Work out the finished part from the listing and answer in its coordinate system (mm). Face numbers are marked on the shaded views. A direction names the side the tool comes from. Coordinates: 2 decimals unless noted, no trailing zeros. Loops run counter-clockwise (first coordinate to the right, second up) from the corner with the lowest first, then second, coordinate; pieces in that order, holes last. Notation, with made-up numbers: (0, 61) - (31, 61) arc R7 cw to (31, 72) - close; hole circle Ø2 at (15.25, 89). An arc over 180 degrees is marked (long way). Write each question's results on one line, items separated by ' | '. Start each with the question number.
Item 1: A tool of negligible diameter and unlimited length cuts with its end or side. For the marked faces 5, 6, 7, 8 and 9, from which of +Z, -Z, +X, -X, +Y, -Y can it reach the whole face along a straight path? Write none if from no direction.
Item 2: Each of these flat-tipped pins is pushed along its axis until it touches: pin 1 Ø2 at (x, y) = (-15.5, 32.5) entering from -Z; pin 2 Ø5.5 at (x, z) = (6.5, -2) entering from +Y; pin 3 Ø2 at (x, y) = (-17, 32) entering from +Z. Where does it stop, or does it pass through?
Item 3: Section A-A, the plane y = 9 is taken. Write down the section's boundary in (x, z), plus the area to 3 significant figures.
Item 4: Consider probe 1 along X at (y, z) = (35, -1.5); probe 2 along X at (y, z) = (-2, 2); probe 3 along Z at (x, y) = (-4.5, -16). Determine where each line is inside the solid, lowest interval first. Write a range as [from, to].
Item 5: For a pull along Y with two mould halves and no side action, classify the marked faces 1, 2, 3 and 4 as +Y half, -Y half, draft (parallel to the pull), parting line (faces both ways), or undercut.
from build123d import *

# Parameters (mm, degrees)
SKETCH2_R           = 3.96875
BOSS_EXTRUDE1_DEPTH = 34.925
CHAMFER2_SIZE       = 1.058333333
SKETCH7_R           = 3.96875
SKETCH9_R           = 3.96875
BOSS_EXTRUDE2_DEPTH = 3.3734375
SKETCH10_OUTSIDE_W  = 257.161
SKETCH10_OUTSIDE_H  = 225.222
SKETCH10_OUTSIDE_R  = 6.35
CUT_EXTRUDE1_DEPTH  = 56.231770933
CUT_EXTRUDE1_TAPER  = 60
SKETCH11_OUTSIDE_W  = 117.847
SKETCH11_OUTSIDE_H  = 85.908
SKETCH11_OUTSIDE_R  = 6.35
CUT_EXTRUDE2_DEPTH  = 16.015104167
CUT_EXTRUDE2_TAPER  = 60
SKETCH12_W          = 52.3875
SKETCH12_H          = 19.05
BOSS_EXTRUDE3_DEPTH = 2.38125


with BuildPart() as part:
    # Sketch2 → Boss-Extrude1 (new body)
    with BuildSketch(Plane(origin=(0, 42.8625, 0), x_dir=(-1, 0, 0), z_dir=(0, 1, 0))):
        with Locations((16.66875, 0)):
            Circle(SKETCH2_R)
    extrude(amount=-BOSS_EXTRUDE1_DEPTH)

    # Chamfer2
    chamfer2_edges = [part.edges().sort_by_distance(p)[0] for p in [
        (-12.7, 42.8625, 0),
    ]]
    chamfer(chamfer2_edges, length=CHAMFER2_SIZE)


with BuildPart() as body_2:
    # Sweep1: sweep along a path in Sketch8
    with BuildLine(Plane.XY) as sweep1_path:
        Line((-16.66875, 7.9375), (-16.66875, 0))
        ThreePointArc((-16.66875, 0), (0, -16.66875), (16.66875, 0))
        Line((16.66875, 0), (16.66875, 7.9375))
    # Sketch7 → Sweep1 (sweep)
    with BuildSketch(Plane(origin=(0, 7.9375, 0), x_dir=(-1, 0, 0), z_dir=(0, 1, 0))):
        with Locations((16.66875, 0)):
            Circle(SKETCH7_R)
    sweep(path=sweep1_path.line)


with BuildPart() as body_3:
    # Body-Move/Copy1: copy of part
    add(part.part.moved(Location((33.3375, 0, 0))))


with BuildPart() as part_1:
    add(part.part)

    # Combine1: union body 2, body 3
    add(body_2.part)
    add(body_3.part)



with BuildPart() as body_2_2:
    # Sketch9 → Boss-Extrude2 (new body, symmetric)
    with BuildSketch(Plane(origin=(0, 31.220833333, 0), x_dir=(-1, 0, 0), z_dir=(0, 1, 0))):
        Polygon((-20.334924209, 6.35), (-24.001098419, 0), (-20.334924209, -6.35), (-13.002575791, -6.35), (-9.336401581, 0), (-13.002575791, 6.35), align=None)
        with Locations((-16.66875, 0)):
            Circle(SKETCH9_R, mode=Mode.SUBTRACT)
    extrude(amount=BOSS_EXTRUDE2_DEPTH, both=True)

    # Sketch10 outside → Cut-Extrude1 (cut, through all)
    with BuildSketch(Plane(origin=(0, 34.594270833, 0), x_dir=(1, 0, 0), z_dir=(0, 1, 0))):
        with Locations((1.6815, 0)):
            Rectangle(SKETCH10_OUTSIDE_W, SKETCH10_OUTSIDE_H)
        with Locations((16.66875, 0)):
            Circle(SKETCH10_OUTSIDE_R, mode=Mode.SUBTRACT)
    extrude(amount=-CUT_EXTRUDE1_DEPTH, taper=CUT_EXTRUDE1_TAPER, mode=Mode.SUBTRACT)

    # Sketch11 outside → Cut-Extrude2 (cut, through all)
    with BuildSketch(Plane.XZ.offset(-27.847395833)):
        with Locations((1.6815, 0)):
            Rectangle(SKETCH11_OUTSIDE_W, SKETCH11_OUTSIDE_H)
        with Locations((16.66875, 0)):
            Circle(SKETCH11_OUTSIDE_R, mode=Mode.SUBTRACT)
    extrude(amount=-CUT_EXTRUDE2_DEPTH, taper=CUT_EXTRUDE2_TAPER, mode=Mode.SUBTRACT)


with BuildPart() as body_3_2:
    # Body-Move/Copy2: copy of body 2 2
    add(body_2_2.part.moved(Location((-33.3375, 0, 0))))


with BuildPart() as part_2:
    add(part_1.part)

    add(body_2_2.part)  # Boss-Extrude3 merges body 2 2

    add(body_3_2.part)  # Boss-Extrude3 merges body 3 2
    # Sketch12 → Boss-Extrude3 (add)
    with BuildSketch(Plane(origin=(0, 27.847395833, 0), x_dir=(1, 0, 0), z_dir=(0, 1, 0))):
        Rectangle(SKETCH12_W, SKETCH12_H)
    extrude(amount=-BOSS_EXTRUDE3_DEPTH)


solid = part_2.part
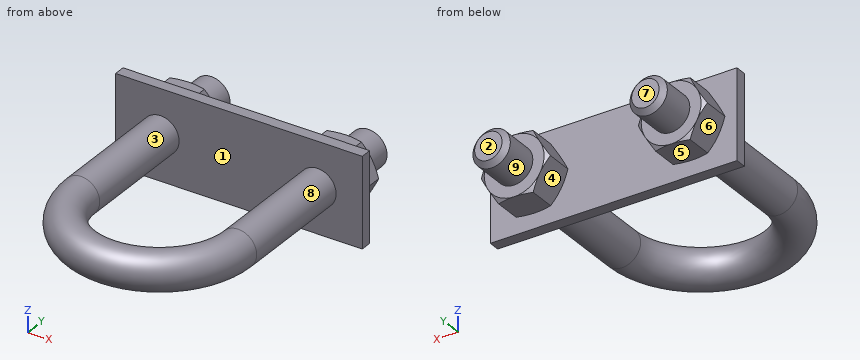
Answer key:
1) face 5: -Z, +X, -X, +Y | face 6: -Z, -X, +Y | face 7: +Z, -Z, +X, -X, +Y | face 8: none | face 9: +Y
2) pin 1: stops at z = -6.35 | pin 2: stops at y = 27.85 | pin 3: stops at z = 6.35
3) outline: circle Ø7.94 at (-16.67, 0); circle Ø7.94 at (16.67, 0) | area: 99.0 mm^2
4) probe 1: x = [-20.34, -12.99], [12.99, 20.34] | probe 2: x = [-20, -13.09], [13.09, 20] | probe 3: z = [-3.97, 3.97]
5) face 1: undercut | face 2: +Y half | face 3: undercut | face 4: draft
